Build history of the part. All positions in model axes, mm. A direction names the side the tool comes from. Round coordinates to 2 decimals unless told otherwise and drop trailing zeros. Write each loop counter-clockwise with the first axis right and the second up, starting at its lowest first coordinate (ties: lowest second). Pieces come first, ordered by that corner, then holes.
from build123d import *

# Parameters (mm, degrees)
BOSS_EXTRUDE1_DEPTH       = 18
CUT_EXTRUDE2_DEPTH        = 43
FILLET2_R                 = 6
SKETCH4_R                 = 4.5
CUT_EXTRUDE3_DEPTH        = 55.0000001
SKETCH5_W                 = 20
SKETCH5_H                 = 20
CUT_EXTRUDE6_DEPTH        = 7.92
CUT_EXTRUDE7_DEPTH        = 12.0000001
F_6_0MM_DOWEL_HOLE1_D     = 6
F_6_0MM_DOWEL_HOLE1_DEPTH = 6
F_6_0MM_DOWEL_HOLE1_TIP   = 1.802581857
CUT_EXTRUDE8_DEPTH        = 43
FILLET3_R                 = 6


with BuildPart() as part:
    # Sketch1 → Boss-Extrude1 (new body, symmetric)
    with BuildSketch(Plane(origin=(0, 0, 0), x_dir=(1, 0, 0), z_dir=(0, 1, 0))):
        with BuildLine():
            Line((19.211898334, 37.921604348), (19.211898334, 40.921604348))
            Line((19.211898334, 40.921604348), (22.211898334, 40.921604348))
            Line((22.211898334, 40.921604348), (22.211898334, 53.921604348))
            Line((22.211898334, 53.921604348), (50.211898334, 53.921604348))
            Line((50.211898334, 53.921604348), (50.211898334, 10.921604348))
            Line((50.211898334, 10.921604348), (79.211898334, 10.921604348))
            Line((79.211898334, 10.921604348), (82.211898334, -0.078395652))
            Line((82.211898334, -0.078395652), (-81.788101666, -0.078395652))
            Line((-81.788101666, -0.078395652), (-78.788101666, 10.921604348))
            Line((-78.788101666, 10.921604348), (-49.788101666, 10.921604348))
            Line((-49.788101666, 10.921604348), (-49.788101666, 53.921604348))
            Line((-49.788101666, 53.921604348), (-21.788101666, 53.921604348))
            Line((-21.788101666, 53.921604348), (-21.788101666, 40.921604348))
            Line((-21.788101666, 40.921604348), (-18.788101666, 40.921604348))
            Line((-18.788101666, 40.921604348), (-18.788101666, 37.921604348))
            ThreePointArc((-18.788101666, 37.921604348), (0.211898334, 18.921604348), (19.211898334, 37.921604348))
        make_face()
    extrude(amount=BOSS_EXTRUDE1_DEPTH, both=True)

    # Sketch3 → Cut-Extrude2 (cut)
    with BuildSketch(Plane(origin=(0, 0, -53.921604348), x_dir=(-1, 0, 0), z_dir=(0, 0, -1))):
        with BuildLine():
            Line((44.497190923, 18), (49.788101666, 18))
            Line((49.788101666, 18), (49.788101666, -18))
            Line((49.788101666, -18), (44.497190923, -18))
            ThreePointArc((44.497190923, -18), (48, 0), (44.497190923, 18))
        make_face()
    extrude(amount=-CUT_EXTRUDE2_DEPTH, mode=Mode.SUBTRACT)

    # Fillet2
    fillet2_edges = [part.edges().sort_by_distance(p)[0] for p in [
        (-48, 0, -10.921604348),
    ]]
    fillet(fillet2_edges, radius=FILLET2_R)

    # Sketch4 → Cut-Extrude3 (cut, through all)
    with BuildSketch(Plane(origin=(0, 0, -53.921604348), x_dir=(-1, 0, 0), z_dir=(0, 0, -1))):
        with Locations((31, 0)):
            Circle(SKETCH4_R)
    cut_extrude3 = extrude(amount=-CUT_EXTRUDE3_DEPTH, mode=Mode.SUBTRACT)

    # Sketch5 → Cut-Extrude6 (cut, symmetric)
    with BuildSketch(Plane.XY):
        with Locations((-31.09995798, -0.141547283)):
            Rectangle(SKETCH5_W, SKETCH5_H)
    cut_extrude6 = extrude(amount=CUT_EXTRUDE6_DEPTH, both=True, mode=Mode.SUBTRACT)

    # Sketch6 → Cut-Extrude7 (cut, through all)
    with BuildSketch(Plane(origin=(0, 0, -10.921604348), x_dir=(-1, 0, 0), z_dir=(0, 0, -1))):
        with BuildLine():
            Line((60, 4), (68, 4))
            ThreePointArc((68, 4), (72, 0), (68, -4))
            Line((68, -4), (60, -4))
            ThreePointArc((60, -4), (56, 0), (60, 4))
        make_face()
    cut_extrude7 = extrude(amount=-CUT_EXTRUDE7_DEPTH, mode=Mode.SUBTRACT)

    # Ø6.0mm Dowel Hole1
    with Locations(Plane(origin=(0, 0, -18.922785988), x_dir=(-0.999937808, 0, -0.011152544), z_dir=(0.011152544, 0, -0.999937808))):
        with Locations((0, 0)):
            Hole(F_6_0MM_DOWEL_HOLE1_D / 2, depth=F_6_0MM_DOWEL_HOLE1_DEPTH)
            with Locations((0, 0, -(F_6_0MM_DOWEL_HOLE1_DEPTH + F_6_0MM_DOWEL_HOLE1_TIP / 2))):  # 118° drill point
                Cone(0, F_6_0MM_DOWEL_HOLE1_D / 2, F_6_0MM_DOWEL_HOLE1_TIP, mode=Mode.SUBTRACT)

    # Mirror3: Cut-Extrude3, Cut-Extrude6, Cut-Extrude7 across plane
    add(cut_extrude3.mirror(Plane(origin=(0, 0, 0), x_dir=(0, 0, 1), z_dir=(1, 0, 0))), mode=Mode.SUBTRACT)
    add(cut_extrude6.mirror(Plane(origin=(0, 0, 0), x_dir=(0, 0, 1), z_dir=(1, 0, 0))), mode=Mode.SUBTRACT)
    add(cut_extrude7.mirror(Plane(origin=(0, 0, 0), x_dir=(0, 0, 1), z_dir=(1, 0, 0))), mode=Mode.SUBTRACT)

    # Sketch10 → Cut-Extrude8 (cut)
    with BuildSketch(Plane(origin=(0, 0, -53.921604348), x_dir=(-1, 0, 0), z_dir=(0, 0, -1))):
        with BuildLine():
            Line((-50.211898334, -18), (-44.410172286, -18))
            ThreePointArc((-44.410172286, -18), (-47.912981363, 0), (-44.410172286, 18))
            Line((-44.410172286, 18), (-50.211898334, 18))
            Line((-50.211898334, 18), (-50.211898334, -18))
        make_face()
    extrude(amount=-CUT_EXTRUDE8_DEPTH, mode=Mode.SUBTRACT)

    # Fillet3
    fillet3_edges = [part.edges().sort_by_distance(p)[0] for p in [
        (47.912981363, 0, -10.921604348),
    ]]
    fillet(fillet3_edges, radius=FILLET3_R)


solid = part.part
1) Slice it at C-C (z = -27). Write the cut outline in (x, y), plus the area to 3 significant figures.
Results:
outline: (-44.5, -18) - (-15.34, -18) - (-15.34, 18) - (-44.5, 18) arc R48 ccw to start; (15.76, -18) - (44.41, -18) arc R48 ccw to (44.41, 18) - (15.76, 18) - close; hole circle Ø9 at (-31, 0); hole circle Ø9 at (31, 0)
area: 2,120 mm2
2) Slice it at B-B (x = 66). Write the cut outline in (y, z).
Results:
outline: (-18, -10.92) - (-4, -10.92) - (-4, 0.08) - (-18, 0.08) - close; (4, -10.92) - (18, -10.92) - (18, 0.08) - (4, 0.08) - close
3) Which spindle directions (+Z, -Z, +X, -X, +Y, -Y) get a long thin tool onto all of the face, cutting with end or side? Do faces 4 (the cylindrical face through (-72, 0, -5)), 5 (the flat face through (21, 0, -40.922)), 6 (the flat face through (31, -10.142, -4)). Say none if no direction does.
Results:
face 4: +Z, -Z
face 5: -Z, +Y, -Y
face 6: +Z
4) Slice it at D-D (x = 31). Write the cut outline in (y, z), plus the area to 3 significant figures.
Results:
outline: (-18, -53.92) - (-4.5, -53.92) - (-4.5, -7.92) - (-10.14, -7.92) - (-10.14, 0.08) - (-18, 0.08) - close; (4.5, -53.92) - (18, -53.92) - (18, 0.08) - (9.86, 0.08) - (9.86, -7.92) - (4.5, -7.92) - close
area: 1,370 mm2
5) Pin check, flat tips, straight feed: pin 1 Ø6.5 at (y, z) = (4, -48.5) entering from -X; pin 2 Ø2 at (x, y) = (13.5, -5) entering from -Z; pin 3 Ø3 at (x, y) = (46.5, 12.5) entering from -Z; pin 4 Ø8.5 at (x, y) = (-59, 3.5) entering from -Z. Stop position of each tip, or through.
Results:
pin 1: stops at x = -47.99
pin 2: stops at z = -25.4
pin 3: stops at z = -53.92
pin 4: stops at z = -10.92
6) Mould opens along X. For faces 1 (the flat face through (80.69, 0.25, -5.5)), 2 (the flat face through (1, -18, -15)), 3 (the flat face through (-36, 0, -7.92)) say: released by +X, released by -X, zero draft, split by the parting line, or undercut.
Results:
face 1: released by +X
face 2: zero draft
face 3: undercut
7) Wall check: L1, parallel to Y at x = -31, z = -44; L2, parallel to X at y = -1.5, z = -52; L3, parallel to Z at x = 19.5, y = -3. Give the ranges that are in metal, low to high.
Results:
L1: y = -18 to -4.5, 4.5 to 18
L2: x = -47.98 to -35.24, -26.76 to -21.79, 22.21 to 26.76, 35.24 to 47.89
L3: z = -40.92 to 0.08
8) Slice it at A-A (z = -46.5). Write the cut outline in (x, y), plus the area to 3 significant figures.
Results:
outline: (-44.5, -18) - (-21.79, -18) - (-21.79, 18) - (-44.5, 18) arc R48 ccw to start; (22.21, -18) - (44.41, -18) arc R48 ccw to (44.41, 18) - (22.21, 18) - close; hole circle Ø9 at (-31, 0); hole circle Ø9 at (31, 0)
area: 1,660 mm2
